Autodesk Inventor part; units mm, degrees
ref_plane "YZ Plane" through (0, 0, 0) normal (1, 0, 0) x (0, 1, 0)
ref_plane "XZ Plane" through (0, 0, 0) normal (0, 1, 0) x (-1, 0, 0)
ref_plane "XY Plane" through (0, 0, 0) normal (0, 0, 1) x (1, 0, 0)
sketch "Sketch1" plane through (0, 0, 0) normal (0, 0, 1) x (1, 0, 0)
  line L0 (-6.35, 3.048) -> (6.35, 3.048)
  line L1 (6.35, 3.048) -> (6.35, -3.048)
  line L2 (6.35, -3.048) -> (-6.35, -3.048)
  line L3 (-6.35, -3.048) -> (-6.35, 3.048)
  point P0 (0, 0)
  point P1 (0, -3.048)
  point P2 (-6.35, 0)
  dimension "d0" = 12.7
  dimension "d1" = 6.096
extrude "Extrusion1" add sketch "Sketch1" along normal blind 15.24
sketch "Sketch2" plane through (-6.35, 3.048, 0) normal (0, 1, 0) x (1, 0, 0)
  line L0 (0, -15.24) -> (12.7, -15.24)
  line L1 (2.54, -13.208) -> (10.16, -13.208)
  line L2 (10.16, -13.208) -> (10.16, -15.24)
  line L3 (10.16, -15.24) -> (2.54, -15.24)
  line L4 (2.54, -15.24) -> (2.54, -13.208)
  point P0 (6.35, -15.24)
  dimension "d4" = 7.62
  dimension "d5" = 2.032
extrude "Extrusion2" add sketch "Sketch2" along normal blind 1.27
sketch "Sketch3" plane through (-6.35, -3.048, 0) normal (0, -1, 0) x (1, 0, 0)
  line L0 (0, 15.24) -> (2.54, 15.24)
  line L1 (2.54, 15.24) -> (2.54, 13.208)
  line L2 (2.54, 13.208) -> (0, 13.208)
  line L3 (0, 13.208) -> (0, 15.24)
  line L4 (12.7, 15.24) -> (10.16, 15.24)
  line L5 (10.16, 15.24) -> (10.16, 13.208)
  line L6 (10.16, 13.208) -> (12.7, 13.208)
  line L7 (12.7, 13.208) -> (12.7, 15.24)
  dimension "d8" = 2.54
  dimension "d9" = 2.54
  dimension "d10" = 2.032
  dimension "d11" = 2.032
extrude "Extrusion3" add sketch "Sketch3" along normal blind 0.508
sketch "Sketch4" plane through (0, 0, 0) normal (0, 0, -1) x (-1, 0, 0)
  line L0 (6.35, 3.048) -> (-6.35, 3.048)
  line L1 (-6.35, 3.048) -> (-6.35, -3.048)
  line L2 (-6.35, -3.048) -> (6.35, -3.048)
  line L3 (6.35, -3.048) -> (6.35, 3.048)
  point P0 (-5.08, 1.27)
  point P1 (-2.54, 1.27)
  point P2 (2.54, 1.27)
  point P3 (5.08, 1.27)
  point P4 (-5.08, -1.27)
  point P5 (-2.54, -1.27)
  point P6 (2.54, -1.27)
  point P7 (5.08, -1.27)
  point P8 (0, 3.048)
  point P9 (0, 1.27)
  point P10 (0, -1.27)
  point P11 (0, 1.27)
  point P12 (0, -1.27)
  dimension "d14" = 1.27
  dimension "d15" = 1.778
  dimension "d16" = 1.27
  dimension "d17" = 1.778
  dimension "d18" = 2.54
  dimension "d19" = 2.54
  dimension "d20" = 2.54
  dimension "d21" = 2.54
properties part number "10 Pin DR"
Here's how the part is built. I have some questions about the finished solid (model axes, mm). A direction names the side the tool comes from. Coordinates: 2 decimals unless noted, no trailing zeros. Write each loop counter-clockwise with the first axis right and the second up, starting at its lowest first coordinate (ties: lowest second). Pieces come first, ordered by that corner, then holes.
1) Which directions (+Z, -Z, +X, -X, +Y, -Y) give clear straight access to the entire face, cutting with the end or side of a thin tool? Please do faces 1 (the face through (-3.81, 4, 14)), 2 (the face through (3.81, 4, 14)), 3 (the face through (0, 4, 13.208)), 4 (the face through (-5, -3.556, 14)).
Filled in:
face 1: +Z, -Z, -X, +Y
face 2: +Z, -Z, +X, +Y
face 3: -Z, +X, -X, +Y
face 4: +Z, -Z, +X, -X, -Y
2) If I drill on line 1 (Y direction, x = 2, z = 10), over which ranges is the centre line in solid material (lowest first)?
Filled in:
line 1: y = -3.05 to 3.05
3) I'm going to push flat-ended pins straight in: pin 1 (0.6 mm diameter, centred on y = 4, z = 14, fed in from +X); pin 2 (1.4 mm diameter, centred on y = 4, z = 14, fed in from -X). Where does each tip first touch, or does it pass through?
Filled in:
pin 1: stops at x = 3.81
pin 2: stops at x = -3.81
4) If we section it at A-A (x = -4.25): List the corners of the cut face in (y, z) for me.
Filled in:
outline: (-3.56, 13.21) - (-3.05, 13.21) - (-3.05, 0) - (3.05, 0) - (3.05, 15.24) - (-3.56, 15.24) - close
5) If we section it at D-D (z = 8): List the corners of the cut face in (x, y) for me.
Filled in:
outline: (-6.35, -3.05) - (6.35, -3.05) - (6.35, 3.05) - (-6.35, 3.05) - close
6) If we section it at B-B (y = 3.25): List the corners of the cut face in (x, z) for me, plus the area to 3 significant figures.
Filled in:
outline: (-3.81, 13.21) - (3.81, 13.21) - (3.81, 15.24) - (-3.81, 15.24) - close
area: 15.5 mm2
7) If we section it at C-C (x = 0): List the corners of the cut face in (y, z) for me.
Filled in:
outline: (-3.05, 0) - (3.05, 0) - (3.05, 13.21) - (4.32, 13.21) - (4.32, 15.24) - (-3.05, 15.24) - close
